Autodesk Inventor part; units mm, degrees
ref_plane "YZ Plane" through (0, 0, 0) normal (1, 0, 0) x (0, 1, 0)
ref_plane "XZ Plane" through (0, 0, 0) normal (0, 1, 0) x (-1, 0, 0)
ref_plane "XY Plane" through (0, 0, 0) normal (0, 0, 1) x (1, 0, 0)
sketch "스케치1" plane through (0, 0, 0) normal (0, 0, 1) x (1, 0, 0)
  circle A0 centre (0, 0) radius 44.5
  line L0 (-42, -42) -> (42, -42)
  line L1 (42, -42) -> (42, 42)
  line L2 (42, 42) -> (-42, 42)
  line L3 (-42, 42) -> (-42, -42)
  line L4 (-42, -42) -> (42, 42) construction
  line L5 (42, -42) -> (-42, 42) construction
  circle A1 centre (0, 0) radius 27.5
  point P0 (-42, 14.7054)
  point P1 (-42, -14.7054)
  point P2 (-14.7054, -42)
  point P3 (14.7054, -42)
  point P4 (42, -14.7054)
  point P5 (42, 14.7054)
  point P6 (14.7054, 42)
  point P7 (-14.7054, 42)
  dimension "d0" = 89
  dimension "d1" = 84
  dimension "d2" = 84
  dimension "d3" = 55
extrude "돌출1" add sketch "스케치1" along normal blind 5 contours L1 A0 L0 L3 L2
sketch "스케치2" plane through (0, 0, 5) normal (0, 0, 1) x (1, 0, 0)
  circle A0 centre (-12, 35) radius 1
  line L0 (0, 0) -> (0, 47.7452)
  circle A1 centre (-12, 35) radius 2
  circle A2 centre (12, 35) radius 1
  circle A3 centre (12, 35) radius 2
  dimension "d6" = 2
  dimension "d7" = 35
  dimension "d8" = 12
  dimension "d9" = 4
extrude "돌출2" cut sketch "스케치2" against normal blind 1.3 contours A0 | A1 | A2 | A3
extrude "돌출3" cut sketch "스케치2" against normal blind 10.5 contours A0 | A2
pattern_circular "원형 패턴1" count 4 over 360 about axis through (0, 0, 0) along (0, 0, 1) of "돌출2", "돌출3"
sketch "스케치3" plane through (0, 0, 5) normal (0, 0, 1) x (1, 0, 0)
  circle A0 centre (0, 0) radius 35 construction
  line L0 (0, 0) -> (-24.7487, 24.7487) construction
  line L1 (0, 0) -> (0, 35) construction
  circle A1 centre (-24.7487, 24.7487) radius 2.25
  dimension "d17" = 70
  dimension "d18" = 45
  dimension "d19" = 4.5
extrude "돌출4" cut sketch "스케치3" against normal blind 5
pattern_circular "원형 패턴2" count 4 over 360 about axis through (0, 0, 0) along (0, 0, 1) of "돌출4"
properties part number "감속기어1 - 하우징 커버"
Read the model definition and answer for the solid it produces. Units are mm, in the model's axes. A direction names the side the tool comes from. Coordinates: 2 decimals unless noted, no trailing zeros. Loops run counter-clockwise (first coordinate to the right, second up) from the corner with the lowest first, then second, coordinate; pieces in that order, holes last. Notation, with made-up numbers: (3, 5.25) -> (34, 5.25) arc R23 ccw to (34, 27.25) -> close; hole circle Ø1 at (81, -8.75). An arc over 180 degrees is marked (long way). Return JSON: item names as keys, results as strings.
Item 1: Find section D-D (y = -35). Determine the outline of the cut face in (x, z).
Answers:
{"outline": "(-27.48, 0) -> (-13, 0) -> (-13, 3.7) -> (-14, 3.7) -> (-14, 5) -> (-27.48, 5) -> close; (-11, 0) -> (11, 0) -> (11, 3.7) -> (10, 3.7) -> (10, 5) -> (-10, 5) -> (-10, 3.7) -> (-11, 3.7) -> close; (13, 0) -> (27.48, 0) -> (27.48, 5) -> (14, 5) -> (14, 3.7) -> (13, 3.7) -> close"}
Item 2: For faces 1 (the cylindrical face through (-5.961, 26.846, 2.465)), 2 (the cylindrical face through (33, -12, 4)), determine the directions among +Z, -Z, +X, -X, +Y, -Y from which every point of the face is accessible in a straight line to the end or side of a thin tool.
Answers:
{"face 1": "+Z, -Z", "face 2": "+Z"}
Item 3: Find the intervals of material crossed by probe 1 along Y at (x, z) = (12, 4); probe 2 along X at (y, z) = (11.5, 3.1); probe 3 along X at (y, z) = (-12, 0.9), in increasing order.
Answers:
{"probe 1": "y = -42 to -37, -33 to -24.74, 24.74 to 33, 37 to 42", "probe 2": "x = -42 to -35.87, -34.13 to -24.98, 24.98 to 34.13, 35.87 to 42", "probe 3": "x = -42 to -36, -34 to -24.74, 24.74 to 34, 36 to 42"}
Item 4: Find section C-C (z = 1.95). Count the separate pieces of the cut face and the enclosed holes in it, plus the area to 3 significant figures.
Answers:
{"separate pieces": "1", "enclosed holes": "13", "area": "3,560 mm2"}
Item 5: Find section A-A (y = 0). Determine the outline of the cut face in (x, z).
Answers:
{"outline": "(-42, 0) -> (-27.5, 0) -> (-27.5, 5) -> (-42, 5) -> close; (27.5, 0) -> (42, 0) -> (42, 5) -> (27.5, 5) -> close"}
Item 6: Flat-ended cylindrical pins translate along their axes: P1, Ø3.5, axis at x = -12, y = -35, coming from the +Z side; P2, Ø6.5, axis at x = -35, y = -12, coming from the +Z side; P3, Ø1.2, axis at x = -35, y = -12, coming from the -Z side; P4, Ø2, axis at x = -16, z = 3.5, coming from the -Y side. Find the tip coordinate at first contact, or state that the pin passes through.
Answers:
{"P1": "stops at z = 3.7", "P2": "stops at z = 5", "P3": "passes through", "P4": "stops at y = -41.9"}
Item 7: For a pull along X with two mould halves and no side action, classify faces 3 (the flat face through (42, 0, 2)), 4 (the cylindrical face through (-31.66, 31.27, 2.46)), 5 (the flat face through (0, 42, 2)), 6 (the cylindrical face through (33, 12, 4)) as +X half, -X half, draft (parallel to the pull), parting line (faces both ways), or undercut.
Answers:
{"face 3": "+X half", "face 4": "-X half", "face 5": "draft", "face 6": "undercut"}
Item 8: Find section B-B (x = 12). Determine the outline of the cut face in (y, z), plus the area to 3 significant figures.
Answers:
{"outline": "(-42, 0) -> (-36, 0) -> (-36, 3.7) -> (-37, 3.7) -> (-37, 5) -> (-42, 5) -> close; (-34, 0) -> (-24.74, 0) -> (-24.74, 5) -> (-33, 5) -> (-33, 3.7) -> (-34, 3.7) -> close; (24.74, 0) -> (34, 0) -> (34, 3.7) -> (33, 3.7) -> (33, 5) -> (24.74, 5) -> close; (36, 0) -> (42, 0) -> (42, 5) -> (37, 5) -> (37, 3.7) -> (36, 3.7) -> close", "area": "147 mm2"}
